```python
from build123d import *

# Parameters (mm, degrees)
SKETCH_1_R          = 43
SKETCH_1_R_2        = 35
EXTRUDE_1_DEPTH     = 4
SKETCH_2_R          = 1.5
CUT_EXTRUDE_1_DEPTH = 10
FILLET_1_R          = 10
FILLET_2_R          = 2
CUT_EXTRUDE_2_DEPTH = 10
FILLET_3_R          = 1.5
SKETCH_4_R          = 1.5
CUT_EXTRUDE_3_DEPTH = 4


with BuildPart() as part:
    # 草图1 → 凸台-拉伸1 (new body)
    # profile 1 of 2: a face of its own
    with BuildSketch(Plane.XY):
        Circle(SKETCH_1_R)
        Circle(SKETCH_1_R_2, mode=Mode.SUBTRACT)
    # profile 2 of 2: a face of its own
    with BuildSketch(Plane.XY):
        with BuildLine():
            ThreePointArc((43, 0), (0, -43), (-43, 0))
            Line((-43, 0), (-43, -40))
            Line((-43, -40), (-60, -40))
            Line((-60, -40), (-60, -65))
            Line((-60, -65), (60, -65))
            Line((60, -65), (60, -40))
            Line((60, -40), (43, -40))
            Line((43, -40), (43, 0))
        make_face()
    extrude(amount=EXTRUDE_1_DEPTH)

    # 草图2 → 切除-拉伸1 (cut)
    with BuildSketch(Plane.XY.offset(4)):
        with Locations((-35, 16.8)):
            Circle(SKETCH_2_R)
        with Locations((-35, -16.8)):
            Circle(SKETCH_2_R)
        with Locations((35, -16.8)):
            Circle(SKETCH_2_R)
        with Locations((35, 16.8)):
            Circle(SKETCH_2_R)
    extrude(amount=-CUT_EXTRUDE_1_DEPTH, mode=Mode.SUBTRACT)

    # 圆角1
    fillet_1_edges = [part.edges().sort_by_distance(p)[0] for p in [
        (43, -40, 2),
        (-43, -40, 2),
    ]]
    fillet(fillet_1_edges, radius=FILLET_1_R)

    # 圆角2
    fillet_2_edges = [part.edges().sort_by_distance(p)[0] for p in [
        (60, -40, 2),
        (60, -65, 2),
        (-60, -65, 2),
        (-60, -40, 2),
    ]]
    fillet(fillet_2_edges, radius=FILLET_2_R)

    # 草图3 → 切除-拉伸2 (cut)
    with BuildSketch(Plane.XY.offset(4)):
        Polygon((-40, -61), (-40, -65), (-20, -65), (-20, -61), (-23, -61), (-37, -61), align=None)
        with BuildLine():
            ThreePointArc((-37, -61), (-38.5, -59.5), (-40, -61))
            Line((-40, -61), (-37, -61))
        make_face()
        with BuildLine():
            Line((-23, -61), (-20, -61))
            ThreePointArc((-20, -61), (-21.5, -59.5), (-23, -61))
        make_face()
        with BuildLine():
            ThreePointArc((3, -61), (1.5, -59.5), (0, -61))
            Line((0, -61), (3, -61))
        make_face()
        Polygon((0, -61), (0, -65), (20, -65), (20, -61), (17, -61), (3, -61), align=None)
        with BuildLine():
            Line((17, -61), (20, -61))
            ThreePointArc((20, -61), (18.5, -59.5), (17, -61))
        make_face()
        with BuildLine():
            ThreePointArc((43, -61), (41.5, -59.5), (40, -61))
            Line((40, -61), (43, -61))
        make_face()
        with BuildLine():
            Line((40, -61), (40, -65))
            Line((40, -65), (58, -65))
            ThreePointArc((58, -65), (59.414213562, -64.414213562), (60, -63))
            Line((60, -63), (60, -61))
            Line((60, -61), (43, -61))
            Line((43, -61), (40, -61))
        make_face()
    extrude(amount=-CUT_EXTRUDE_2_DEPTH, mode=Mode.SUBTRACT)

    # 圆角3
    fillet_3_edges = [part.edges().sort_by_distance(p)[0] for p in [
        (60, -61, 2),
    ]]
    fillet(fillet_3_edges, radius=FILLET_3_R)

    # 草图4 → 切除-拉伸3 (cut)
    with BuildSketch(Plane(origin=(0, 0, 0), x_dir=(-1, 0, 0), z_dir=(0, 0, -1))):
        with Locations((-55, -58)):
            Circle(SKETCH_4_R)
        with Locations((-35, -58)):
            Circle(SKETCH_4_R)
        with Locations((-15, -58)):
            Circle(SKETCH_4_R)
        with Locations((5, -58)):
            Circle(SKETCH_4_R)
        with Locations((25, -58)):
            Circle(SKETCH_4_R)
        with Locations((45, -58)):
            Circle(SKETCH_4_R)
    extrude(amount=-CUT_EXTRUDE_3_DEPTH, mode=Mode.SUBTRACT)


solid = part.part
```
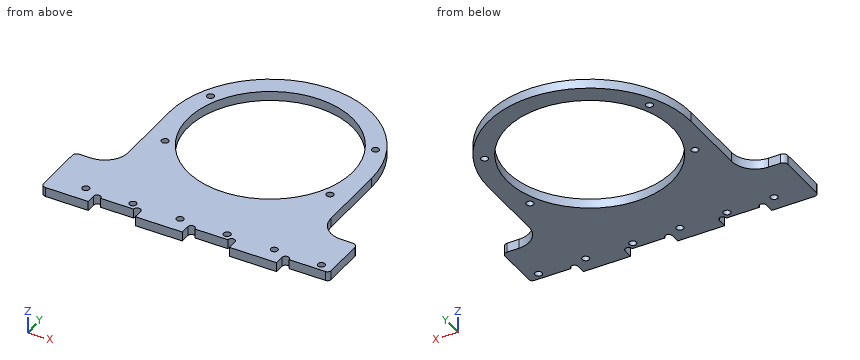
Source: CAD feature listing. Evaluate the final solid. Frame: model axes, mm. Round coordinates to 2 decimals unless told otherwise and drop trailing zeros. Loops run counter-clockwise (first coordinate to the right, second up) from the corner with the lowest first, then second, coordinate; pieces in that order, holes last. Notation, with made-up numbers: M 43.25,-29.5 L 84.25,-29.5 A20 cw 84.25,-25.5 Z; hole C -16.5,14.5 d8. An arc over 180 degrees is marked long. Use a Markdown table: item, result. Add a question column.
1. Ray query, line 1 along Y through (x, z) = (15, 2.7); line 2 along Y through (x, z) = (-25.5, 2.9); line 3 along Y through (x, z) = (19, 1.2). Return the intervals inside material, ascending. Write a range as [from, to].
2. Cut plane B-B, the plane x = -21.5. Output: boundary loops of the cut face in (y, z).
3. Cut plane A-A, the plane y = -58. Output: boundary loops of the cut face in (x, z).
4. Cut plane D-D, the plane x = 15. Output: boundary loops of the cut face in (y, z), and give its area (3 significant figures).
5. Cut plane C-C, the plane y = -21. Output: boundary loops of the cut face in (x, z), and give its area (3 significant figures).
6. Contact query for flat-ended pins moving along their axis: pin 1 (2 mm diameter, centred on y = -15, z = 3, fed in from +X); pin 2 (2 mm diameter, centred on y = -5.5, z = 2.5, fed in from -X); pin 3 (1.2 mm diameter, centred on x = -54.5, z = 2.5, fed in from +Y). Output: stop coordinate, or through.
Solution:
| question | item | result |
|---|---|---|
| 1 | line 1 | y = [-61, -59.5], [-56.5, -31.62], [31.62, 40.3] |
| 1 | line 2 | y = [-61, -59.41], [-56.59, -23.97], [23.97, 34.62] |
| 1 | line 3 | y = [-59.59, -29.39], [29.39, 38.57] |
| 2 | outline | M -59.5,0 L -27.62,0 L -27.62,4 L -59.5,4 Z; M 27.62,0 L 37.24,0 L 37.24,4 L 27.62,4 Z |
| 3 | outline | M -60,0 L -46.5,0 L -46.5,4 L -60,4 Z; M -43.5,0 L -26.5,0 L -26.5,4 L -43.5,4 Z; M -23.5,0 L -6.5,0 L -6.5,4 L -23.5,4 Z; M -3.5,0 L 13.5,0 L 13.5,4 L -3.5,4 Z; M 16.5,0 L 33.5,0 L 33.5,4 L 16.5,4 Z; M 36.5,0 L 53.5,0 L 53.5,4 L 36.5,4 Z; M 56.5,0 L 60,0 L 60,4 L 56.5,4 Z |
| 4 | outline | M -61,0 L -59.5,0 L -59.5,4 L -61,4 Z; M -56.5,0 L -31.62,0 L -31.62,4 L -56.5,4 Z; M 31.62,0 L 40.3,0 L 40.3,4 L 31.62,4 Z |
| 4 | area | 140 mm2 |
| 5 | outline | M -43,0 L -28,0 L -28,4 L -43,4 Z; M 28,0 L 43,0 L 43,4 L 28,4 Z |
| 5 | area | 120 mm2 |
| 6 | pin 1 | stops at x = 43 |
| 6 | pin 2 | stops at x = -43 |
| 6 | pin 3 | stops at y = -40 |
